Verification items for the finished model (mm, model axes). A direction names the side the tool comes from. Coordinates: 2 decimals unless noted, no trailing zeros. Order: outer loops, then holes, each group sorted by start corner. A loop starts at its lowest first (then second) coordinate and runs counter-clockwise, first axis right, second up. Notation, with made-up numbers: M 44,6.5 L 98,6.5 A20 ccw 98,29.5 Z; hole C 1,-16.5 d10. An arc over 180 degrees is marked long. Write item = value, one per line.
```python
from build123d import *

# Parameters (mm, degrees)
FILLET005_R = 1
FILLET006_R = 1
FILLET007_R = 1
FILLET008_R = 0.2
FILLET009_R = 0.2


with BuildPart() as part:
    # Sketch006 → Revolution003 (revolve)
    with BuildSketch(Plane.XZ):
        Polygon((-1.654667, 64.072456), (-9.586614, 64.072456), (-9.586614, 65.072456), (-6.501082, 68.157988), (-5.452098, 68.157988), (-5.452098, 65.502701), (-3.250405, 65.502701), (-3.250405, 67.098916), (-1.654667, 67.098916), align=None)
    revolve(axis=Axis((0, 0, 0), (0, 0, 1)))

    # Fillet005
    fillet005_edges = [part.edges().sort_by_distance(p)[0] for p in [
        (6.501082, 0, 68.157988),
    ]]
    fillet(fillet005_edges, radius=FILLET005_R)

    # Fillet006
    fillet006_edges = [part.edges().sort_by_distance(p)[0] for p in [
        (9.586614, 0, 65.072456),
    ]]
    fillet(fillet006_edges, radius=FILLET006_R)

    # Fillet007
    fillet007_edges = [part.edges().sort_by_distance(p)[0] for p in [
        (1.654667, 0, 67.098916),
    ]]
    fillet(fillet007_edges, radius=FILLET007_R)

    # Fillet008
    fillet008_edges = [part.edges().sort_by_distance(p)[0] for p in [
        (5.452098, 0, 68.157988),
    ]]
    fillet(fillet008_edges, radius=FILLET008_R)

    # Fillet009
    fillet009_edges = [part.edges().sort_by_distance(p)[0] for p in [
        (3.250405, 0, 67.098916),
    ]]
    fillet(fillet009_edges, radius=FILLET009_R)


solid = part.part
```
Item 1: Release check for a two-part mould opening along Y. For faces 3 (the cylindrical face through (-5.2, -1.64, 66.71)), 4 (the flat face through (0, 2, 64.072)), 5 (the conical face through (5.49, 4.21, 67.74)) record: pulls with the +Y half, pulls with the -Y half, needs draft (parallel to the pull), parting line crosses it, or undercut.
Report:
face_3 = undercut
face_4 = needs draft
face_5 = parting line crosses it
Item 2: Gauge pin test, flat ends, axial feed: pin 1 (6.5 mm diameter, centred on x = 1.5, y = 1, fed in from +Z); pin 2 (10 mm diameter, centred on x = 6, y = 4, fed in from +Z); pin 3 (1.5 mm diameter, centred on x = 3, z = 67, fed in from +Y). Record the tip position at first contact, or that the pin passes through.
Report:
pin_1 = 67.1
pin_2 = 68.16
pin_3 = 7.9
Item 3: Scan lines: L1, parallel to Y at x = 0, z = 66.55; L2, parallel to X at y = 0, z = 64.5; L3, parallel to Y at x = 0, z = 65.7. Record each from-to range of solid material in increasing order. Write a range as from..to.
Report:
L1 = -8.11..-5.45, -3.25..-1.76, 1.76..3.25, 5.45..8.11
L2 = -9.59..-1.65, 1.65..9.59
L3 = -8.96..-5.45, -3.25..-1.65, 1.65..3.25, 5.45..8.96
Item 4: Sectioned sample at A-A, the plane z = 64.4. Enter the section's corners in (x, y).
Report:
outline = C 0,0 d19.17; hole C 0,0 d3.31
Item 5: Tool access check on faces 1 (the cylindrical face through (0.705, 3.173, 66.211)), 2 (the cylindrical face through (0.359, 1.615, 65.072)). Record the directions out of +Z, -Z, +X, -X, +Y, -Y that give a thin tool (end or side, any length) a straight path to the whole face; none if there is none.
Report:
face_1 = +Z
face_2 = +Z, -Z
